Geometry: final body of the model. Coordinates: model frame, mm. A direction names the side the tool comes from. Give positions to 0.01 mm unless a question says otherwise; leave off trailing zeros. Loops run counter-clockwise (first coordinate to the right, second up) from the corner with the lowest first, then second, coordinate; pieces in that order, holes last. Notation, with made-up numbers: (83.5, -6.75) - (99.5, -6.75) arc R7 ccw to (99.5, 3.25) - close; hole circle Ø10 at (-38.5, 73.5). An arc over 180 degrees is marked (long way). Use one line per item in the form item = value.
```python
from build123d import *

# Parameters (mm, degrees)
SKETCH_1_W          = 16
SKETCH_1_H          = 7
EXTRUDE_1_DEPTH     = 15.5
CUT_EXTRUDE_1_DEPTH = 7.5
M3X0_51_AT_2_COUNT  = 2
M3X0_51_AT_2_PITCH  = 10


with BuildPart() as part:
    # Эскиз1 → Бобышка-Вытянуть1 (new body)
    with BuildSketch(Plane(origin=(0, 0, 0), x_dir=(1, 0, 0), z_dir=(0, 1, 0))):
        with Locations((8, 3.5)):
            Rectangle(SKETCH_1_W, SKETCH_1_H)
    extrude(amount=EXTRUDE_1_DEPTH)

    # Эскиз2 → Вырез-Вытянуть1 (cut)
    with BuildSketch(Plane(origin=(0, 15.5, 0), x_dir=(1, 0, 0), z_dir=(0, 1, 0))):
        Polygon((-40.166209025, -17.929810867), (0, 0.8), (6.862422146, 4), (14, 4), (16, 2), (47.337917628, -29.337917628), (58.796749642, 58.555289271), (-28.70737701, 69.963396032), align=None)
    extrude(amount=-CUT_EXTRUDE_1_DEPTH, mode=Mode.SUBTRACT)

    # Эскиз3 → Отверстие обработанное метчиком M3x0.51 (revolve, cut)
    with BuildSketch(Plane(origin=(3, 4, -7), x_dir=(0, 1, 0), z_dir=(1, 0, 0))):
        Polygon((0, 0), (0, 7), (1.6, 7), (1.5, 6.9), (1.5, 0.1), (1.6, 0), align=None)
    m3x0_51 = revolve(axis=Axis((3, 4, -13.35), (0, 0, 1)), mode=Mode.SUBTRACT)

    # Отверстие обработанное метчиком M3x0.51 at 2: Отверстие обработанное метчиком M3x0.51 ×2
    with Locations(*[(i * M3X0_51_AT_2_PITCH, 0, 0) for i in range(1, M3X0_51_AT_2_COUNT)]):
        add(m3x0_51, mode=Mode.SUBTRACT)


solid = part.part
```
(1) Pull-direction query (X, two-part tool) for faces 4 (the face through (3.383, 11.802, -2.378)), 5 (the face through (2.55, 5.43, -3.55)), 6 (the face through (6, 8, -5)); classes: released by +X, released by -X, zero draft, split by the parting line, or undercut.
Solution:
face_4 = released by -X
face_5 = undercut
face_6 = zero draft
(2) Cut plane C-C (z = -4.25). Return the cut outline in (x, y).
Solution:
outline = (0, 0) - (16, 0) - (16, 8) - (0, 8) - close; hole circle Ø3 at (3, 4); hole circle Ø3 at (13, 4)
(3) Cut plane D-D (y = 13). Return the cut outline in (x, z), plus the area to 3 significant figures.
Solution:
outline = (0, -0.8) - (6.86, -4) - (14, -4) - (16, -2) - (16, 0) - (0, 0) - close
area = 51.0 mm2
(4) Access query for faces 1 (the face through (10, 12, -4)), 2 (the face through (0, 4, -3)), 3 (the face through (15, 12, -3)). Directions: +Z, -Z, +X, -X, +Y, -Y. A direction counts if a zero-diameter tool reaches every point of the face in a straight line with its end or side. Return the directions, or none.
Solution:
face_1 = -Z, +X, -X, +Y
face_2 = +Z, -Z, -X, +Y, -Y
face_3 = -Z, +X, +Y
(5) Material intervals for L1, parallel to X at y = 4, z = -3.25; L2, parallel to Y at x = 13, z = -4.5; L3, parallel to X at y = 3.5, z = -6.25, sorted ascending. Write a range as from..to.
Solution:
L1 = 0..1.5, 4.5..11.5, 14.5..16
L2 = 0..2.5, 5.5..8
L3 = 0..1.59, 4.41..11.59, 14.41..16
(6) Cut plane A-A (x = 13). Return the cut outline in (y, z), plus the area to 3 significant figures.
Solution:
outline = (0, -7) - (2.4, -7) - (2.5, -6.9) - (2.5, -0.1) - (2.4, 0) - (0, 0) - close; (5.5, -6.9) - (5.6, -7) - (8, -7) - (8, -4) - (15.5, -4) - (15.5, 0) - (5.6, 0) - (5.5, -0.1) - close
area = 65.0 mm2
(7) Cut plane B-B (y = 4). Return the cut outline in (x, z).
Solution:
outline = (0, -7) - (1.4, -7) - (1.5, -6.9) - (1.5, -0.1) - (1.4, 0) - (0, 0) - close; (4.5, -6.9) - (4.6, -7) - (11.4, -7) - (11.5, -6.9) - (11.5, -0.1) - (11.4, 0) - (4.6, 0) - (4.5, -0.1) - close; (14.5, -6.9) - (14.6, -7) - (16, -7) - (16, 0) - (14.6, 0) - (14.5, -0.1) - close
(8) Pin query (flat end, axial travel): P1, Ø2, axis at x = 9, y = 13, coming from the -Z side; P2, Ø1.9, axis at x = 5.5, z = -5, coming from the +Y side; P3, Ø1.8, axis at x = 3, y = 4, coming from the +Z side. Return the tip coordinate at first contact, or that it passes through.
Solution:
P1 = -4
P2 = 8
P3 = through
